Source: CAD feature listing. Evaluate the final solid. Frame: model axes, mm. A direction names the side the tool comes from. Coordinates: 2 decimals unless noted, no trailing zeros. Order: outer loops, then holes, each group sorted by start corner. A loop starts at its lowest first (then second) coordinate and runs counter-clockwise, first axis right, second up.
```python
from build123d import *

# Parameters (mm, degrees)
BOSS_EXTRUDE1_DEPTH = 299.72


with BuildPart() as part:
    # Sketch1 → Boss-Extrude1 (new body)
    with BuildSketch(Plane(origin=(0, 0, 0), x_dir=(1, 0, 0), z_dir=(0, 1, 0))):
        with BuildLine():
            Line((158.75, 0), (184.15, 0))
            ThreePointArc((184.15, 0), (0, 184.15), (-184.15, 0))
            Line((-184.15, 0), (-158.75, 0))
            ThreePointArc((-158.75, 0), (-162.304954792, 8.812386064), (-170.97962963, 12.691286448))
            ThreePointArc((-170.97962963, 12.691286448), (-169.983221483, 22.378715656), (-168.438386668, 31.993943123))
            ThreePointArc((-168.438386668, 31.993943123), (-153.340724923, 41.08752341), (-161.868893389, 56.511625822))
            ThreePointArc((-161.868893389, 56.511625822), (-158.399145849, 65.611074479), (-154.418346013, 74.498838344))
            ThreePointArc((-154.418346013, 74.498838344), (-137.481532851, 79.375), (-141.727059565, 96.480791286))
            ThreePointArc((-141.727059565, 96.480791286), (-136.020430193, 104.372147004), (-129.874950266, 111.926760846))
            ThreePointArc((-129.874950266, 111.926760846), (-112.253201513, 112.253201513), (-111.926760846, 129.874950266))
            ThreePointArc((-111.926760846, 129.874950266), (-104.372147004, 136.020430193), (-96.480791286, 141.727059565))
            ThreePointArc((-96.480791286, 141.727059565), (-79.375, 137.481532851), (-74.498838344, 154.418346013))
            ThreePointArc((-74.498838344, 154.418346013), (-65.611074479, 158.399145849), (-56.511625822, 161.868893389))
            ThreePointArc((-56.511625822, 161.868893389), (-41.08752341, 153.340724923), (-31.993943123, 168.438386668))
            ThreePointArc((-31.993943123, 168.438386668), (-22.378715656, 169.983221483), (-12.691286448, 170.97962963))
            ThreePointArc((-12.691286448, 170.97962963), (0, 158.75), (12.691286448, 170.97962963))
            ThreePointArc((12.691286448, 170.97962963), (22.378715656, 169.983221483), (31.993943123, 168.438386668))
            ThreePointArc((31.993943123, 168.438386668), (41.08752341, 153.340724923), (56.511625822, 161.868893389))
            ThreePointArc((56.511625822, 161.868893389), (65.611074479, 158.399145849), (74.498838344, 154.418346013))
            ThreePointArc((74.498838344, 154.418346013), (79.375, 137.481532851), (96.480791286, 141.727059565))
            ThreePointArc((96.480791286, 141.727059565), (104.372147004, 136.020430193), (111.926760846, 129.874950266))
            ThreePointArc((111.926760846, 129.874950266), (112.253201513, 112.253201513), (129.874950266, 111.926760846))
            ThreePointArc((129.874950266, 111.926760846), (136.020430193, 104.372147004), (141.727059565, 96.480791286))
            ThreePointArc((141.727059565, 96.480791286), (137.481532851, 79.375), (154.418346013, 74.498838344))
            ThreePointArc((154.418346013, 74.498838344), (158.399145849, 65.611074479), (161.868893389, 56.511625822))
            ThreePointArc((161.868893389, 56.511625822), (153.340724923, 41.08752341), (168.438386668, 31.993943123))
            ThreePointArc((168.438386668, 31.993943123), (169.983221483, 22.378715656), (170.97962963, 12.691286448))
            ThreePointArc((170.97962963, 12.691286448), (162.304954792, 8.812386064), (158.75, 0))
        make_face()
    extrude(amount=-BOSS_EXTRUDE1_DEPTH)


solid = part.part
```
1. Contact query for flat-ended pins moving along their axis: P1, Ø1.5, axis at y = -267.5, z = -142, coming from the -X side; P2, Ø8, axis at y = -189.5, z = -105, coming from the -X side; P3, Ø12, axis at y = -133.5, z = -74, coming from the -X side. Output: stop coordinate, or through.
2. Material intervals for line 1 along X through (y, z) = (-86, -163); line 2 along X through (y, z) = (-270.5, -105); line 3 along X through (y, z) = (-69, -132), sorted ascending.
3. Section query C-C, the plane x = 0. Output: boundary loops of the cut face in (y, z), plus the area to 3 significant figures.
4. Section query A-A, the plane z = -62. Output: boundary loops of the cut face in (x, y).
5. Section query B-B, the plane y = -41. Output: boundary loops of the cut face in (x, z) (3 decimals).
6. Access query for faces 4 (the cylindrical face through (-136.103, -147.762, -104.264)), 5 (the flat face through (171, -148, 0)). Directions: +Z, -Z, +X, -X, +Y, -Y. A direction counts if a zero-diameter tool reaches every point of the face in a straight line with its end or side. Return the directions, or none.
7. Section query D-D, the plane z = -88.5. Output: boundary loops of the cut face in (x, y).
8. Draft query along X for faces 1 (the cylindrical face through (4.049, -147.762, -184.105)), 2 (the flat face through (-172, -148, 0)), 3 (the cylindrical face through (-65.737, -147.762, -158.347)). Return one class per face: +X half, -X half, draft (parallel to the pull), parting line (faces both ways), or undercut.
Answer key:
1. P1: stops at x = -118.15
1. P2: stops at x = -153.98
1. P3: stops at x = -171.14
2. line 1: x = -85.69 to -31.95, -9.48 to 9.48, 31.95 to 85.69
2. line 2: x = -151.28 to -135.54, 135.54 to 151.28
2. line 3: x = -128.4 to -109.41, 109.41 to 128.4
3. outline: (-299.72, -184.15) - (0, -184.15) - (0, -158.75) - (-299.72, -158.75) - close
3. area: 7,610 mm2
4. outline: (-173.4, -299.72) - (-159.85, -299.72) - (-159.85, 0) - (-173.4, 0) - close; (159.85, -299.72) - (173.4, -299.72) - (173.4, 0) - (159.85, 0) - close
5. outline: (-184.15, 0) arc R184.15 ccw to (184.15, 0) - (158.75, 0) arc R12.7 ccw to (170.98, -12.691) arc R171.45 cw to (168.438, -31.994) arc R12.7 ccw to (161.869, -56.512) arc R171.45 cw to (154.418, -74.499) arc R12.7 ccw to (141.727, -96.481) arc R171.45 cw to (129.875, -111.927) arc R12.7 ccw to (111.927, -129.875) arc R171.45 cw to (96.481, -141.727) arc R12.7 ccw to (74.499, -154.418) arc R171.45 cw to (56.512, -161.869) arc R12.7 ccw to (31.994, -168.438) arc R171.45 cw to (12.691, -170.98) arc R12.7 ccw to (-12.691, -170.98) arc R171.45 cw to (-31.994, -168.438) arc R12.7 ccw to (-56.512, -161.869) arc R171.45 cw to (-74.499, -154.418) arc R12.7 ccw to (-96.481, -141.727) arc R171.45 cw to (-111.927, -129.875) arc R12.7 ccw to (-129.875, -111.927) arc R171.45 cw to (-141.727, -96.481) arc R12.7 ccw to (-154.418, -74.499) arc R171.45 cw to (-161.869, -56.512) arc R12.7 ccw to (-168.438, -31.994) arc R171.45 cw to (-170.98, -12.691) arc R12.7 ccw to (-158.75, 0) - close
6. face 4: +Y, -Y
6. face 5: +Z, +X, -X, +Y, -Y
7. outline: (-161.49, -299.72) - (-136.09, -299.72) - (-136.09, 0) - (-161.49, 0) - close; (136.09, -299.72) - (161.49, -299.72) - (161.49, 0) - (136.09, 0) - close
8. face 1: parting line
8. face 2: draft
8. face 3: undercut
